Could you check a few things on this model? Use its own coordinates, in mm. A direction names the side the tool comes from. Coordinates: 2 decimals unless noted, no trailing zeros. Loops run counter-clockwise (first coordinate to the right, second up) from the corner with the lowest first, then second, coordinate; pieces in that order, holes last. Notation, with made-up numbers: (-33, 23) - (-4, 23) arc R33 cw to (-4, 62) - close; hole circle Ø8 at (-18, 1). An arc over 180 degrees is marked (long way). One line per item, written item: value. Start each with the question number.
(1) If we section it at C-C on x = 0.25: Write out the boundary of the cut face in (y, z), then the cut area to 3 significant figures.
(2) On a 3-axis mill with a long thin cutter (end or side, diameter ignored), from which of +Z, -Z, +X, -X, +Y, -Y can I reach the whole of each face in a straight line? I mean faces 1 (the face through (-4.25, -0.09, 5.07)), 2 (the face through (0, -7.1, 6)). Say none if no direction works.
(3) If we section it at A-A on z = 5.5: Write out the boundary of the cut face in (x, y), then the cut area to 3 significant figures.
(4) If we mould it in two halves opening along Y, with no side actions, what happens to faces 3 (the face through (3.05, -0.09, 6.06)), 4 (the face through (0, 0, 0)), 5 (the face through (0, 8.3, 5))? For each: pulls with the +Y half, pulls with the -Y half, needs draft (parallel to the pull), parting line crosses it, or undercut.
(5) If we section it at D-D on x = -3.5: Write out the boundary of the cut face in (y, z), then the cut area to 3 significant figures.
(6) I'm going to push flat-ended pins straight in: P1, Ø4, axis at y = -2, z = 5, coming from the +X side; P2, Ø2, axis at y = -1, z = 2, coming from the -X side; P3, Ø1.5, axis at y = -2.5, z = 6, coming from the -X side. Where does each tip first touch, or does it pass through?
(7) If we section it at B-B on z = 1.5: Write out the boundary of the cut face in (x, y), then the cut area to 3 significant figures.
(8) If I drill on line 1 along Y through (x, z) = (2, 6); line 2 along Z through (x, y) = (2.25, -5); line 3 along X through (y, z) = (0.25, 4), over which ranges is the centre line in solid material (lowest first)? Write a range as from..to.
```python
from build123d import *

# Parameters (mm, degrees)
F0_W     = 14
F0_H     = 20
F1_DEPTH = 10
F3_DEPTH = 8
F4_R     = 0.5
F5_W     = 14
F5_H     = 20
F6_DEPTH = 10


with BuildPart() as f1:
    # F0 (on Top) → F1 (new body)
    with BuildSketch(Plane.XY):
        Rectangle(F0_W, F0_H)
    extrude(amount=F1_DEPTH)

    # F2 (on face) → F3 (cut)
    with BuildSketch(Plane.XY.offset(10)):
        with BuildLine():
            ThreePointArc((3.9, -7.1), (3.05, 0), (3.9, 7.1))
            Line((3.9, 7.1), (-3.9, 7.1))
            ThreePointArc((-3.9, 7.1), (-3.2632560046, 3.5753496333), (-3.05, 0))
            ThreePointArc((-3.05, 0), (-3.2632560046, -3.5753496333), (-3.9, -7.1))
            Line((-3.9, -7.1), (3.9, -7.1))
        make_face()
    extrude(amount=-F3_DEPTH, mode=Mode.SUBTRACT)

    # F4
    f4_edges = [f1.edges().sort_by_distance(p)[0] for p in [
        (-3.9, 7.1, 6),
        (-3.9, -7.1, 6),
        (3.9, 7.1, 6),
        (3.9, -7.1, 6),
    ]]
    fillet(f4_edges, radius=F4_R)

    # F5 (on face) → F6 (cut, through all)
    with BuildSketch(Plane.XY.offset(10)):
        Rectangle(F5_W, F5_H)
        with BuildLine():
            ThreePointArc((4.9307012466, -6.2330688212), (4.5962509216, -7.6644756916), (3.2707730825, -8.3))
            Line((3.2707730825, -8.3), (-3.2707730825, -8.3))
            ThreePointArc((-3.2707730825, -8.3), (-4.5962509216, -7.6644756916), (-4.9307012466, -6.2330688212))
            ThreePointArc((-4.9307012466, -6.2330688212), (-4.25, 0), (-4.9307012466, 6.2330688212))
            ThreePointArc((-4.9307012466, 6.2330688212), (-4.5962509216, 7.6644756916), (-3.2707730825, 8.3))
            Line((-3.2707730825, 8.3), (3.2707730825, 8.3))
            ThreePointArc((3.2707730825, 8.3), (4.5962509216, 7.6644756916), (4.9307012466, 6.2330688212))
            ThreePointArc((4.9307012466, 6.2330688212), (4.25, 0), (4.9307012466, -6.2330688212))
        make_face(mode=Mode.SUBTRACT)
    extrude(amount=-F6_DEPTH, mode=Mode.SUBTRACT)


solid = f1.part
```
Values:
1. outline: (-8.3, 0) - (8.3, 0) - (8.3, 10) - (7.1, 10) - (7.1, 2) - (-7.1, 2) - (-7.1, 10) - (-8.3, 10) - close
1. area: 52.4 mm2
2. face 1: +Z, -Z, -X
2. face 2: +Z
3. outline: (-4.93, -6.23) arc R1.7 ccw to (-3.27, -8.3) - (3.27, -8.3) arc R1.7 ccw to (4.93, -6.23) arc R28.88 cw to (4.93, 6.23) arc R1.7 ccw to (3.27, 8.3) - (-3.27, 8.3) arc R1.7 ccw to (-4.93, 6.23) arc R28.88 cw to start; hole (-3.76, -6.49) arc R0.5 ccw to (-3.27, -7.1) - (3.27, -7.1) arc R0.5 ccw to (3.76, -6.49) arc R30.08 cw to (3.76, 6.49) arc R0.5 ccw to (3.27, 7.1) - (-3.27, 7.1) arc R0.5 ccw to (-3.76, 6.49) arc R30.08 cw to start
3. area: 55.9 mm2
4. face 3: undercut
4. face 4: needs draft
4. face 5: pulls with the +Y half
5. outline: (-8.28, 0) - (8.28, 0) - (8.28, 10) - (7.04, 10) - (7.04, 2) - (5.18, 2) - (5.18, 10) - (-5.18, 10) - (-5.18, 2) - (-7.04, 2) - (-7.04, 10) - (-8.28, 10) - close
5. area: 136 mm2
6. P1: stops at x = 4.53
6. P2: stops at x = -4.32
6. P3: stops at x = -4.43
7. outline: (-4.93, -6.23) arc R1.7 ccw to (-3.27, -8.3) - (3.27, -8.3) arc R1.7 ccw to (4.93, -6.23) arc R28.88 cw to (4.93, 6.23) arc R1.7 ccw to (3.27, 8.3) - (-3.27, 8.3) arc R1.7 ccw to (-4.93, 6.23) arc R28.88 cw to start
7. area: 150 mm2
8. line 1: y = -8.3..-7.1, 7.1..8.3
8. line 2: z = 0..2
8. line 3: x = -4.25..-3.05, 3.05..4.25
